Could you check a few things on this model? Use its own coordinates, in mm. Face numbers are marked on the shaded views. A direction names the side the tool comes from. Round coordinates to 2 decimals unless told otherwise and drop trailing zeros. Loops run counter-clockwise (first coordinate to the right, second up) from the corner with the lowest first, then second, coordinate; pieces in that order, holes last. Notation, with made-up numbers: (63.25, 4) - (74.25, 4) arc R37 cw to (74.25, 43) - close; hole circle Ø1 at (23, 51). An arc over 180 degrees is marked (long way). Put each result on its own line as item: value. Start each with the question number.
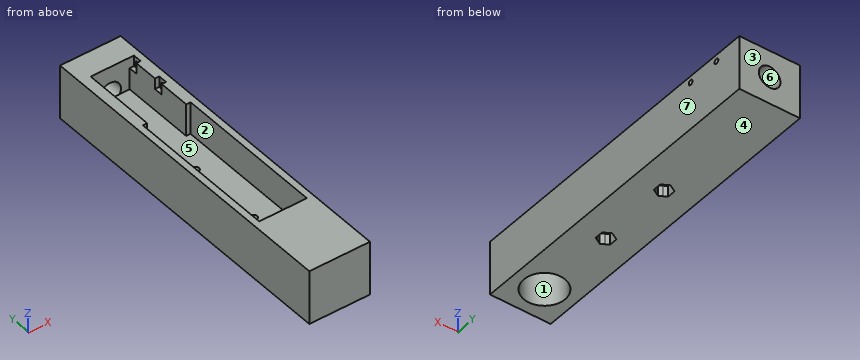
from build123d import *

# Parameters (mm, degrees)
F0_W      = 28
F0_H      = 25
F1_DEPTH  = 150
F2_R      = 9.525
F3_DEPTH  = 17
F4_R      = 1.5
F5_DEPTH  = 5
F6_R      = 1.5
F7_DEPTH  = 25.001
F8_W      = 22
F8_H      = 70
F9_DEPTH  = 15
F10_R     = 1.15
F11_DEPTH = 5
F12_W     = 2
F12_H     = 4.0241825168
F13_DEPTH = 5
F14_W     = 18
F14_H     = 19.2723592291
F15_DEPTH = 15
F16_W     = 18
F16_H     = 14.7685540254
F17_DEPTH = 15
F18_R     = 5
F19_DEPTH = 12


# Not quite as in the source:
# - the program builds the solid bodies; features that only make, move or delete a surface that nothing else refers to are left out


with BuildPart() as f1:
    # F0 (on Front) → F1 (new body)
    with BuildSketch(Plane.XZ):
        Rectangle(F0_W, F0_H)
    extrude(amount=-F1_DEPTH)

    # F2 (on face) → F3 (cut)
    with BuildSketch(Plane(origin=(0, 0, -12.5), x_dir=(1, 0, 0), z_dir=(0, 0, -1))):
        with Locations((0, -14.525)):
            Circle(F2_R)
    extrude(amount=-F3_DEPTH, mode=Mode.SUBTRACT)

    # F4 (on face) → F5 (cut)
    with BuildSketch(Plane(origin=(0, 0, -12.5), x_dir=(1, 0, 0), z_dir=(0, 0, -1))):
        with BuildLine():
            ThreePointArc((1.6602502077, -54.4256372334), (2.8756374132, -53.2102498962), (3.3205, -51.55))
            ThreePointArc((3.3205, -51.55), (2.8756373339, -49.8897499664), (1.6602499328, -48.6743626079))
            ThreePointArc((1.6602499328, -48.6743626079), (-1.397e-07, -48.2295), (-1.6602501748, -48.6743627476))
            ThreePointArc((-1.6602501748, -48.6743627476), (-2.8756374037, -49.8897500874), (-3.3205, -51.55))
            ThreePointArc((-3.3205, -51.55), (-2.8756373712, -53.210249969), (-1.660250062, -54.4256373175))
            ThreePointArc((-1.660250062, -54.4256373175), (8.41e-08, -54.8705), (1.6602502077, -54.4256372334))
        make_face()
        with Locations((0, -51.55)):
            Circle(F4_R, mode=Mode.SUBTRACT)
        with BuildLine():
            Line((3.3205, -53.4670915688), (3.3205, -51.55))
            ThreePointArc((3.3205, -51.55), (2.8756374132, -53.2102498962), (1.6602502077, -54.4256372334))
            Line((1.6602502077, -54.4256372334), (3.3205, -53.4670915688))
        make_face()
        with BuildLine():
            ThreePointArc((1.6602499328, -48.6743626079), (2.8756373339, -49.8897499664), (3.3205, -51.55))
            Line((3.3205, -51.55), (3.3205, -49.6329084312))
            Line((3.3205, -49.6329084312), (1.6602499328, -48.6743626079))
        make_face()
        with BuildLine():
            ThreePointArc((-1.6602501748, -48.6743627476), (-1.397e-07, -48.2295), (1.6602499328, -48.6743626079))
            Line((1.6602499328, -48.6743626079), (0, -47.7158168623))
            Line((0, -47.7158168623), (-1.6602501748, -48.6743627476))
        make_face()
        with BuildLine():
            Line((0, -55.3841831377), (1.6602502077, -54.4256372334))
            ThreePointArc((1.6602502077, -54.4256372334), (8.41e-08, -54.8705), (-1.660250062, -54.4256373175))
            Line((-1.660250062, -54.4256373175), (0, -55.3841831377))
        make_face()
        with BuildLine():
            ThreePointArc((-3.3205, -51.55), (-2.8756374037, -49.8897500874), (-1.6602501748, -48.6743627476))
            Line((-1.6602501748, -48.6743627476), (-3.3205, -49.6329084312))
            Line((-3.3205, -49.6329084312), (-3.3205, -51.55))
        make_face()
        with BuildLine():
            Line((-3.3205, -53.4670915688), (-1.660250062, -54.4256373175))
            ThreePointArc((-1.660250062, -54.4256373175), (-2.8756373712, -53.210249969), (-3.3205, -51.55))
            Line((-3.3205, -51.55), (-3.3205, -53.4670915688))
        make_face()
        with BuildLine():
            ThreePointArc((1.6602500198, -89.4256373418), (2.875637359, -88.2102499901), (3.3205, -86.55))
            ThreePointArc((3.3205, -86.55), (2.8756374351, -84.8897501418), (1.6602502837, -83.6743628105))
            ThreePointArc((1.6602502837, -83.6743628105), (-2.2e-09, -83.2295), (-1.6602502875, -83.6743628127))
            ThreePointArc((-1.6602502875, -83.6743628127), (-2.8756374363, -84.8897501438), (-3.3205, -86.55))
            ThreePointArc((-3.3205, -86.55), (-2.875637359, -88.2102499901), (-1.6602500198, -89.4256373418))
            ThreePointArc((-1.6602500198, -89.4256373418), (0, -89.8705), (1.6602500198, -89.4256373418))
        make_face()
        with Locations((0, -86.55)):
            Circle(F4_R, mode=Mode.SUBTRACT)
        with BuildLine():
            Line((3.3205, -88.4670915688), (3.3205, -86.55))
            ThreePointArc((3.3205, -86.55), (2.875637359, -88.2102499901), (1.6602500198, -89.4256373418))
            Line((1.6602500198, -89.4256373418), (3.3205, -88.4670915688))
        make_face()
        with BuildLine():
            ThreePointArc((1.6602502837, -83.6743628105), (2.8756374351, -84.8897501418), (3.3205, -86.55))
            Line((3.3205, -86.55), (3.3205, -84.6329084312))
            Line((3.3205, -84.6329084312), (1.6602502837, -83.6743628105))
        make_face()
        with BuildLine():
            ThreePointArc((-1.6602502875, -83.6743628127), (-2.2e-09, -83.2295), (1.6602502837, -83.6743628105))
            Line((1.6602502837, -83.6743628105), (0, -82.7158168623))
            Line((0, -82.7158168623), (-1.6602502875, -83.6743628127))
        make_face()
        with BuildLine():
            Line((0, -90.3841831377), (1.6602500198, -89.4256373418))
            ThreePointArc((1.6602500198, -89.4256373418), (0, -89.8705), (-1.6602500198, -89.4256373418))
            Line((-1.6602500198, -89.4256373418), (0, -90.3841831377))
        make_face()
        with BuildLine():
            ThreePointArc((-3.3205, -86.55), (-2.8756374363, -84.8897501438), (-1.6602502875, -83.6743628127))
            Line((-1.6602502875, -83.6743628127), (-3.3205, -84.6329084312))
            Line((-3.3205, -84.6329084312), (-3.3205, -86.55))
        make_face()
        with BuildLine():
            Line((-3.3205, -88.4670915688), (-1.6602500198, -89.4256373418))
            ThreePointArc((-1.6602500198, -89.4256373418), (-2.875637359, -88.2102499901), (-3.3205, -86.55))
            Line((-3.3205, -86.55), (-3.3205, -88.4670915688))
        make_face()
    extrude(amount=-F5_DEPTH, mode=Mode.SUBTRACT)

    # F6 (on face) → F7 (cut, through all)
    with BuildSketch(Plane(origin=(0, 0, -12.5), x_dir=(1, 0, 0), z_dir=(0, 0, -1))):
        with Locations((0, -51.55)):
            Circle(F6_R)
        with Locations((0, -86.55)):
            Circle(F6_R)
    extrude(amount=-F7_DEPTH, mode=Mode.SUBTRACT)

    # F8 (on face) → F9 (cut)
    with BuildSketch(Plane.XY.offset(12.5)):
        with Locations((0, 69.05)):
            Rectangle(F8_W, F8_H)
    extrude(amount=-F9_DEPTH, mode=Mode.SUBTRACT)

    # F10 (on face) → F11 (cut)
    with BuildSketch(Plane.YZ.offset(14)):
        with Locations((136.2115726471, 9.5113839224)):
            Circle(F10_R)
        with Locations((120.7115726471, 9.5113839224)):
            Circle(F10_R)
    extrude(amount=-F11_DEPTH, mode=Mode.SUBTRACT)

    # F12 (on face) → F13 (cut)
    with BuildSketch(Plane.XY.offset(12.5)):
        with Locations((10, 120.8306452838)):
            Rectangle(F12_W, F12_H)
        with Locations((10, 136.0788219961)):
            Rectangle(F12_W, F12_H)
    extrude(amount=-F13_DEPTH, mode=Mode.SUBTRACT)

    # F14 (on face) → F15 (cut)
    with BuildSketch(Plane.XY.offset(12.5)):
        with Locations((0, 128.45473364)):
            Rectangle(F14_W, F14_H)
    extrude(amount=-F15_DEPTH, mode=Mode.SUBTRACT)

    # F16 (on face) → F17 (cut)
    with BuildSketch(Plane.XY.offset(12.5)):
        with Locations((0, 111.4342770127)):
            Rectangle(F16_W, F16_H)
    extrude(amount=-F17_DEPTH, mode=Mode.SUBTRACT)

    # F18 (on face) → F19 (cut)
    with BuildSketch(Plane(origin=(0, 150, 0), x_dir=(-1, 0, 0), z_dir=(0, 1, 0))):
        Circle(F18_R)
    extrude(amount=-F19_DEPTH, mode=Mode.SUBTRACT)


solid = f1.part
Item 1: Thinking about a two-plate mould opening in X: for the marked faces 4, 5, 6 and 7, which applies, released by +X, released by -X, zero draft, split by the parting line, or undercut?
Item 2: I need wall thicknesses on line 1 (Y direction, x = -2.75, z = 6.5); line 2 (X direction, y = 51.55, z = -5.35); line 3 (X direction, y = 109.5, z = 6.5). Which ranges of each line are inside material? Lowest first, please. Write a range as from..to.
Item 3: Suppose I cut it at A-A, the plane y = 51.55. List the corners of the cut face in (x, z) for me, then the cut area to 3 significant figures.
Item 4: On a 3-axis mill with a long thin cutter (end or side, diameter ignored), from which of +Z, -Z, +X, -X, +Y, -Y can I reach the whole of each face in a straight line? I mean the marked faces 1, 2 and 3. Say none if no direction works.
Item 5: Suppose I cut it at D-D, the plane z = 0. List the corners of the cut face in (x, y) for me (3 decimals), then the cut area to 3 significant figures.
Item 6: Suppose I cut it at B-B, the plane y = 96.5. List the corners of the cut face in (x, z) for me.
Item 7: Will this pin go through, and if not, where does the flat tip stop? P1, Ø12, axis at x = 0, y = 52, coming from the +Z side.
Item 8: Suppose I cut it at C-C, the plane z = -8.75. Count the separate pieces of the cut face and the enclosed holes in it, then the cut area to 3 significant figures.
Numbers:
1. face 4: zero draft
1. face 5: undercut
1. face 6: undercut
1. face 7: released by +X
2. line 1: 0..34.05, 138.09..150
2. line 2: -14..-1.5, 1.5..14
2. line 3: -14..-9, 9..14
3. outline: (-14, -12.5) - (-3.32, -12.5) - (-3.32, -7.5) - (-1.5, -7.5) - (-1.5, -2.5) - (-11, -2.5) - (-11, 12.5) - (-14, 12.5) - close; (1.5, -7.5) - (3.32, -7.5) - (3.32, -12.5) - (14, -12.5) - (14, 12.5) - (11, 12.5) - (11, -2.5) - (1.5, -2.5) - close
3. area: 322 mm^2
4. face 1: -Z
4. face 2: +Z
4. face 3: +Z, -Z, +X, -X, +Y
5. outline: (-14, 0) - (14, 0) - (14, 150) - (5, 150) - (5, 138.091) - (9, 138.091) - (9, 104.05) - (11, 104.05) - (11, 34.05) - (-11, 34.05) - (-11, 104.05) - (-9, 104.05) - (-9, 138.091) - (-5, 138.091) - (-5, 150) - (-14, 150) - close; hole circle Ø19.05 at (0, 14.525)
5. area: 1,640 mm^2
6. outline: (-14, -12.5) - (14, -12.5) - (14, 12.5) - (11, 12.5) - (11, -2.5) - (-11, -2.5) - (-11, 12.5) - (-14, 12.5) - close
7. P1: z = -2.5
8. separate pieces: 1
8. enclosed holes: 3
8. area: 3,840 mm^2
